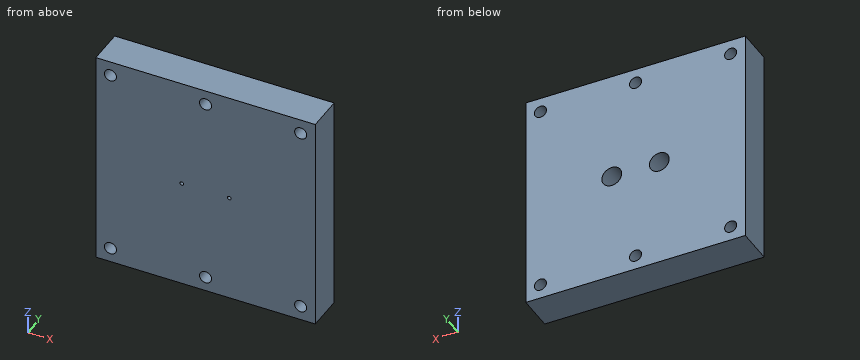
from build123d import *

# Parameters (mm, degrees)
SKETCH2_W                       = 60
SKETCH2_H                       = 60
BOSS_EXTRUDE1_DEPTH             = 10
TAP_DRILL_FOR_M4X0_7_TAP1_D     = 3.3
TAP_DRILL_FOR_M4X0_7_TAP1_DEPTH = 10
F_1_4_28_TAPPED_HOLE5_D         = 5.4102
F_1_4_28_TAPPED_HOLE5_DEPTH     = 7
F_1_4_28_TAPPED_HOLE5_TIP       = 1.625388061
F_1_0MM_DOWEL_HOLE1_D           = 1


with BuildPart() as part:
    # Sketch2 → Boss-Extrude1 (new body)
    with BuildSketch(Plane(origin=(0, 0, 0), x_dir=(1, 0, 0), z_dir=(0, 1, 0))):
        Rectangle(SKETCH2_W, SKETCH2_H)
    extrude(amount=BOSS_EXTRUDE1_DEPTH)

    # Tap Drill for M4x0.7 Tap1
    with Locations(Plane(origin=(0, 0, 0), x_dir=(-1, 0, 0), z_dir=(0, -1, 0))):
        with Locations((0, 26), (26, 26), (-26, 26), (-26, -26), (0, -26), (26, -26)):
            Hole(TAP_DRILL_FOR_M4X0_7_TAP1_D / 2, depth=TAP_DRILL_FOR_M4X0_7_TAP1_DEPTH)

    # 1/4-28 Tapped Hole5
    with Locations(Plane(origin=(0, 10, 0), x_dir=(-1, 0, 0), z_dir=(0, 1, 0))):
        with Locations((6.5, 0), (-6.5, 0)):
            Hole(F_1_4_28_TAPPED_HOLE5_D / 2, depth=F_1_4_28_TAPPED_HOLE5_DEPTH)
            with Locations((0, 0, -(F_1_4_28_TAPPED_HOLE5_DEPTH + F_1_4_28_TAPPED_HOLE5_TIP / 2))):  # 118° drill point
                Cone(0, F_1_4_28_TAPPED_HOLE5_D / 2, F_1_4_28_TAPPED_HOLE5_TIP, mode=Mode.SUBTRACT)

    # Ø1.0mm Dowel Hole1 (through all)
    with Locations(Plane(origin=(0, 10, 0), x_dir=(1, 0, 0), z_dir=(0, 1, 0))):
        with Locations((-6.5, 0), (6.5, 0)):
            Hole(F_1_0MM_DOWEL_HOLE1_D / 2)


solid = part.part
Build history of the part. All positions in model axes, mm. Give positions to 0.01 mm unless a question says otherwise; leave off trailing zeros. Order: outer loops, then holes, each group sorted by start corner. A loop starts at its lowest first (then second) coordinate and runs counter-clockwise, first axis right, second up. Notation, with made-up numbers: M 62.25,37 L 73.25,37 A14 cw 73.25,41 Z; hole C 20.5,23.25 d2. An arc over 180 degrees is marked long. Put each result on its own line as item: value.
Item 1: Cut at C-C on x = -0.5. Write the cut outline in (y, z).
Results are:
outline: M 0,-30 L 10,-30 L 10,-27.57 L 0,-27.57 Z; M 0,-24.43 L 10,-24.43 L 10,24.43 L 0,24.43 Z; M 0,27.57 L 10,27.57 L 10,30 L 0,30 Z
Item 2: Cut at B-B on x = -26. Write the cut outline in (y, z).
Results are:
outline: M 0,-30 L 10,-30 L 10,-27.65 L 0,-27.65 Z; M 0,-24.35 L 10,-24.35 L 10,24.35 L 0,24.35 Z; M 0,27.65 L 10,27.65 L 10,30 L 0,30 Z
Item 3: Drop a flat-ended pin along its axis: pin 1 Ø3 at (x, z) = (26, 26) entering from -Y. Give the stop position or say it passes through.
Results are:
pin 1: through
Item 4: Cut at A-A on y = 4. Count the separate pieces of the cut face and the enclosed holes in it, then the cut area to 3 significant figures.
Results are:
separate pieces: 1
enclosed holes: 8
area: 3,500 mm2
Item 5: Wall check: probe 1 along Z at (x, y) = (-26, 5.25); probe 2 along X at (y, z) = (2.5, -26); probe 3 along X at (y, z) = (7, 0). Give the ranges that are in metal, low to high.
Results are:
probe 1: -30 to -27.65, -24.35 to 24.35, 27.65 to 30
probe 2: -30 to -27.65, -24.35 to -1.65, 1.65 to 24.35, 27.65 to 30
probe 3: -30 to -9.21, -3.79 to 3.79, 9.21 to 30
